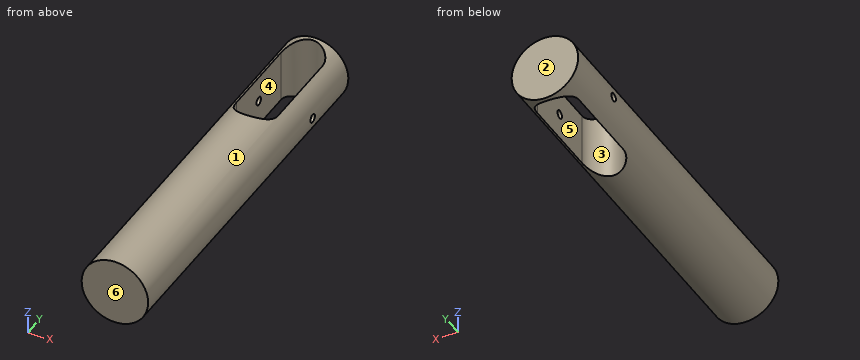
```python
from build123d import *

# Parameters (mm, degrees)
SKETCH1_R               = 40
BOSS_EXTRUDE1_DEPTH     = 450
CUT_EXTRUDE1_DEPTH      = 454.541618818
CUT_EXTRUDE1_DEPTH_BACK = 454.541618818
CUT_EXTRUDE2_DEPTH      = 454.541618935
CUT_EXTRUDE2_DEPTH_BACK = 454.541618935
SKETCH3_R               = 5


with BuildPart() as part:
    # Sketch1 → Boss-Extrude1 (new body)
    with BuildSketch(Plane(origin=(0, 0, 0), x_dir=(1, 0, 0), z_dir=(0, 1, 0))):
        with Locations(Location((0, 0, 0), (0, 0, 270))):
            Circle(SKETCH1_R)
    extrude(amount=BOSS_EXTRUDE1_DEPTH)

    # Sketch2 → Cut-Extrude1 (cut, two sides: drawn at the far end of the back side and taken through both)
    with BuildSketch(Plane.XY.offset(-CUT_EXTRUDE1_DEPTH_BACK)):
        with BuildLine():
            Line((25, 420), (25, 320))
            ThreePointArc((25, 320), (0, 295), (-25, 320))
            Line((-25, 320), (-25, 420))
            ThreePointArc((-25, 420), (0, 445), (25, 420))
        make_face()
    extrude(amount=CUT_EXTRUDE1_DEPTH + CUT_EXTRUDE1_DEPTH_BACK, mode=Mode.SUBTRACT)

    # Sketch3 → Cut-Extrude2 (cut, two sides: drawn at the far end of the back side and taken through both)
    with BuildSketch(Plane(origin=(0, 0, 0), x_dir=(0, 0, -1), z_dir=(1, 0, 0)).offset(-CUT_EXTRUDE2_DEPTH_BACK)):
        with Locations((0, 370)):
            Circle(SKETCH3_R)
    extrude(amount=CUT_EXTRUDE2_DEPTH + CUT_EXTRUDE2_DEPTH_BACK, mode=Mode.SUBTRACT)


solid = part.part
```
Source: CAD feature listing. Evaluate the final solid. Frame: model axes, mm. Face numbers are marked on the shaded views. A direction names the side the tool comes from. Give positions to 0.01 mm unless a question says otherwise; leave off trailing zeros. Order: outer loops, then holes, each group sorted by start corner. A loop starts at its lowest first (then second) coordinate and runs counter-clockwise, first axis right, second up.
(1) Contact query for flat-ended pins moving along their axis: P1, Ø1, axis at y = 326.5, z = -15, coming from the -X side; P2, Ø10, axis at y = 370, z = -14.5, coming from the -X side; P3, Ø6, axis at y = 68, z = 1, coming from the -X side. Output: stop coordinate, or through.
(2) Section query C-C (y = 370). Return the cut outline in (x, z).
(3) Section query D-D (z = 23.5). Return the cut outline in (x, y).
(4) Section query A-A (x = 0). Return the cut outline in (y, z).
(5) Material intervals for line 1 along Y through (x, z) = (32.5, 0); line 2 along X through (y, z) = (347.5, -2.5); line 3 along X through (y, z) = (180, 2), sorted ascending.
(6) Section query B-B (z = 0). Return the cut outline in (x, y).
(7) Pull-direction query (X, two-part tool) for the marked faces 1, 2, 3 and 4; classes: +X half, -X half, draft (parallel to the pull), parting line (faces both ways), or undercut.
(8) Access query for the marked faces 5 and 6. Directions: +Z, -Z, +X, -X, +Y, -Y. A direction counts if a zero-diameter tool reaches every point of the face in a straight line with its end or side. Return the directions, or none.
Outcome:
1. P1: stops at x = -37.28
1. P2: stops at x = -38.86
1. P3: stops at x = -40
2. outline: (-39.69, -5) arc R40 ccw to (-25, -31.22) - (-25, -5) - close; (-39.69, 5) - (-25, 5) - (-25, 31.22) arc R40 ccw to start; (25, -31.22) arc R40 ccw to (39.69, -5) - (25, -5) - close; (25, 5) - (39.69, 5) arc R40 ccw to (25, 31.22) - close
3. outline: (-32.37, 0) - (32.37, 0) - (32.37, 450) - (-32.37, 450) - close; hole (-25, 320) arc R25 ccw to (25, 320) - (25, 420) arc R25 ccw to (-25, 420) - close
4. outline: (0, -40) - (295, -40) - (295, 40) - (0, 40) - close; (445, -40) - (450, -40) - (450, 40) - (445, 40) - close
5. line 1: y = 0 to 365, 375 to 450
5. line 2: x = -39.92 to -25, 25 to 39.92
5. line 3: x = -39.95 to 39.95
6. outline: (-40, 0) - (40, 0) - (40, 365) - (25, 365) - (25, 320) arc R25 cw to (-25, 320) - (-25, 365) - (-40, 365) - close; (-40, 375) - (-25, 375) - (-25, 420) arc R25 cw to (25, 420) - (25, 375) - (40, 375) - (40, 450) - (-40, 450) - close
7. face 1: parting line
7. face 2: draft
7. face 3: undercut
7. face 4: undercut
8. face 5: +Z, -Z
8. face 6: +Z, -Z, +X, -X, -Y
